Source: CAD feature listing. Evaluate the final solid. Frame: model axes, mm. Face numbers are marked on the shaded views. A direction names the side the tool comes from. Give positions to 0.01 mm unless a question says otherwise; leave off trailing zeros. Loops run counter-clockwise (first coordinate to the right, second up) from the corner with the lowest first, then second, coordinate; pieces in that order, holes last. Notation, with made-up numbers: M 7,37 L 29,37 A15 cw 29,55 Z; hole C 72,76 d1. An arc over 180 degrees is marked long. Write item = value, one per line.
from build123d import *

# Parameters (mm, degrees)
F0_R     = 6.35
F1_DEPTH = 16.002
F2_R     = 9.652
F3_W     = 76.2
F3_H     = 28.448
F4_DEPTH = 16.002
F5_R     = 9.652
F6_R     = 14.224
F8_DEPTH = 16.003


with BuildPart() as f1:
    # F0 (on Front) → F1 (new body)
    with BuildSketch(Plane.XZ):
        with BuildLine():
            ThreePointArc((25.4, 44.45), (12.7, 57.15), (0, 44.45))
            Line((0, 44.45), (0, 0))
            Line((0, 0), (101.6, 0))
            Line((101.6, 0), (101.6, 44.45))
            ThreePointArc((101.6, 44.45), (88.9, 57.15), (76.2, 44.45))
            Line((76.2, 44.45), (76.2, 16.002))
            Line((76.2, 16.002), (25.4, 16.002))
            Line((25.4, 16.002), (25.4, 44.45))
        make_face()
        with Locations((12.7, 44.45)):
            Circle(F0_R, mode=Mode.SUBTRACT)
        with Locations((88.9, 44.45)):
            Circle(F0_R, mode=Mode.SUBTRACT)
    extrude(amount=F1_DEPTH)

    # F2
    f2_edges = [f1.edges().sort_by_distance(p)[0] for p in [
        (25.4, -8.001, 16.002),
        (76.2, -8.001, 16.002),
    ]]
    fillet(f2_edges, radius=F2_R)

    # F3 (on Top) → F4 (join)
    with BuildSketch(Plane.XY):
        with Locations((50.8, -30.226)):
            Rectangle(F3_W, F3_H)
    extrude(amount=F4_DEPTH)

    # F5
    f5_edges = [f1.edges().sort_by_distance(p)[0] for p in [
        (12.7, -16.002, 8.001),
        (88.9, -16.002, 8.001),
    ]]
    fillet(f5_edges, radius=F5_R)

    # F6
    f6_edges = [f1.edges().sort_by_distance(p)[0] for p in [
        (12.7, -44.45, 8.001),
        (88.9, -44.45, 8.001),
    ]]
    fillet(f6_edges, radius=F6_R)

    # F7 (on face) → F8 (cut, through all)
    with BuildSketch(Plane.XY.offset(16.002)):
        with BuildLine():
            Line((69.85, -25.4), (31.75, -25.4))
            ThreePointArc((31.75, -25.4), (25.4, -31.75), (31.75, -38.1))
            Line((31.75, -38.1), (69.85, -38.1))
            ThreePointArc((69.85, -38.1), (76.2, -31.75), (69.85, -25.4))
        make_face()
    extrude(amount=-F8_DEPTH, mode=Mode.SUBTRACT)


solid = f1.part
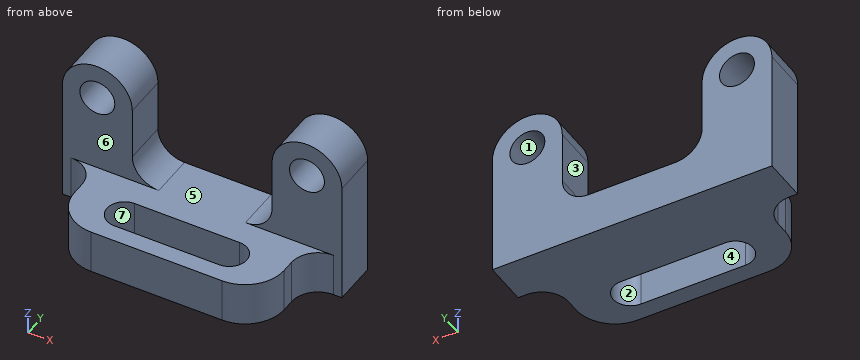
1. Cut plane A-A, the plane z = 29. Return the cut outline in (x, y).
Derived:
outline = M 0,-16 L 25.4,-16 L 25.4,0 L 0,0 Z; M 76.2,-16 L 101.6,-16 L 101.6,0 L 76.2,0 Z
2. Cut plane C-C, the plane y = -15. Return the cut outline in (x, z).
Derived:
outline = M 0,0 L 101.6,0 L 101.6,44.45 A12.7 ccw 76.2,44.45 L 76.2,25.65 A9.65 cw 66.55,16 L 35.05,16 A9.65 cw 25.4,25.65 L 25.4,44.45 A12.7 ccw 0,44.45 Z; hole C 12.7,44.45 d12.7; hole C 88.9,44.45 d12.7
3. Cut plane B-B, the plane x = 54.5. Return the cut outline in (y, z).
Derived:
outline = M -44.45,0 L -38.1,0 L -38.1,16 L -44.45,16 Z; M -25.4,0 L 0,0 L 0,16 L -25.4,16 Z
4. Reachability of the marked faces 1, 2 and 3 from +Z, -Z, +X, -X, +Y, -Y: full face, straight path, thin tool, end or side. Return the list, or none.
Derived:
face_1 = +Y, -Y
face_2 = +Z, -Z
face_3 = +Z, +Y, -Y
5. Cut plane D-D, the plane z = 8.5. Return the cut outline in (x, y).
Derived:
outline = M 0,-16 L 3.05,-16 A9.65 cw 12.7,-25.65 L 12.7,-30.23 A14.22 ccw 26.92,-44.45 L 74.68,-44.45 A14.22 ccw 88.9,-30.23 L 88.9,-25.65 A9.65 cw 98.55,-16 L 101.6,-16 L 101.6,0 L 0,0 Z; hole M 31.75,-38.1 L 69.85,-38.1 A6.35 ccw 69.85,-25.4 L 31.75,-25.4 A6.35 ccw Z
6. First-contact query: pin 1 Ø2.5 at (y, z) = (-27, 7.5) entering from +X; pin 2 Ø4 at (x, y) = (89, -26.5) entering from +Z; pin 3 Ø10.5 at (x, z) = (79, 18) entering from -Y; pin 4 Ø10 at (x, z) = (85.5, 22) entering from -Y. Flat tips, straight axial feed; report the tip coordinate or a pass-through.
Derived:
pin_1 = 88.9
pin_2 = 16
pin_3 = -44.45
pin_4 = -16
7. Material intervals for probe 1 along Y at (x, z) = (50, 14); probe 2 along Z at (x, y) = (88.9, -8); probe 3 along Z at (x, y) = (50, -15), sorted ascending. Write a range as from..to.
Derived:
probe_1 = -44.45..-38.1, -25.4..0
probe_2 = 0..38.1, 50.8..57.15
probe_3 = 0..16
8. Pull-direction query (Y, two-part tool) for the marked faces 4, 5, 6 and 7; classes: +Y half, -Y half, draft (parallel to the pull), parting line (faces both ways), or undercut.
Derived:
face_4 = undercut
face_5 = draft
face_6 = -Y half
face_7 = undercut
